from build123d import *

# Parameters (mm, degrees)
SKETCH_1_W             = 90
SKETCH_1_H             = 70
SKETCH_1_R             = 5.5
SKETCH_1_R_2           = 2.5
SM_BASE_FLANGE_1_DEPTH = 2


# Sheet-metal steps are written as plain solids
with BuildPart() as part:
    # Sketch 1 → Базовая кромка1 (new body)
    with BuildSketch(Plane.XY):
        with Locations((45, 35)):
            Rectangle(SKETCH_1_W, SKETCH_1_H)
        with Locations((45, 35)):
            Circle(SKETCH_1_R, mode=Mode.SUBTRACT)
        with Locations((10, 60)):
            Circle(SKETCH_1_R_2, mode=Mode.SUBTRACT)
        with Locations((80, 60)):
            Circle(SKETCH_1_R_2, mode=Mode.SUBTRACT)
        with Locations((10, 5)):
            Circle(SKETCH_1_R_2, mode=Mode.SUBTRACT)
        with Locations((80, 5)):
            Circle(SKETCH_1_R_2, mode=Mode.SUBTRACT)
    extrude(amount=-SM_BASE_FLANGE_1_DEPTH)


solid = part.part
Geometry check sheet. Reference: the model listing, model coordinates, mm. Round coordinates to 2 decimals unless told otherwise and drop trailing zeros. Order: outer loops, then holes, each group sorted by start corner. A loop starts at its lowest first (then second) coordinate and runs counter-clockwise, first axis right, second up. Notation, with made-up numbers: M 74,35 L 97,35 A24 cw 97,62 Z; hole C 84,1.25 d4. An arc over 180 degrees is marked long. Answer in a Markdown table with one row per item. Add a question column.
Item 1: Material ranges on L1, parallel to Y at x = 80, z = -0.8; L2, parallel to Y at x = 44.5, z = -0.15; L3, parallel to X at y = 5.5, z = -1.6, recorded low to high. Write a range as [from, to].
Item 2: Sectioned sample at C-C, the plane z = -0.7. Enter the section's corners in (x, y), plus the area to 3 significant figures.
Item 3: Sectioned sample at B-B, the plane y = 5. Enter the section's corners in (x, z).
Item 4: Sectioned sample at A-A, the plane x = 45. Enter the section's corners in (y, z).
Item 5: Draft check along X on faces 1 (the face through (0, 35, -1)), 2 (the face through (77.5, 5.1, -1)), 3 (the face through (44, 70, -1)). Enter one of: released by +X, released by -X, zero draft, split by the parting line, or undercut.
Item 6: Sectioned sample at D-D, the plane x = 80. Enter the section's corners in (y, z).
Filled in:
| question | item | result |
|---|---|---|
| 1 | L1 | y = [0, 2.5], [7.5, 57.5], [62.5, 70] |
| 1 | L2 | y = [0, 29.52], [40.48, 70] |
| 1 | L3 | x = [0, 7.55], [12.45, 77.55], [82.45, 90] |
| 2 | outline | M 0,0 L 90,0 L 90,70 L 0,70 Z; hole C 10,5 d5; hole C 10,60 d5; hole C 45,35 d11; hole C 80,5 d5; hole C 80,60 d5 |
| 2 | area | 6,130 mm² |
| 3 | outline | M 0,-2 L 7.5,-2 L 7.5,0 L 0,0 Z; M 12.5,-2 L 77.5,-2 L 77.5,0 L 12.5,0 Z; M 82.5,-2 L 90,-2 L 90,0 L 82.5,0 Z |
| 4 | outline | M 0,-2 L 29.5,-2 L 29.5,0 L 0,0 Z; M 40.5,-2 L 70,-2 L 70,0 L 40.5,0 Z |
| 5 | face 1 | released by -X |
| 5 | face 2 | undercut |
| 5 | face 3 | zero draft |
| 6 | outline | M 0,-2 L 2.5,-2 L 2.5,0 L 0,0 Z; M 7.5,-2 L 57.5,-2 L 57.5,0 L 7.5,0 Z; M 62.5,-2 L 70,-2 L 70,0 L 62.5,0 Z |
